```python
from build123d import *

# Parameters (mm, degrees)
BOSS_EXTRUDE1_DEPTH = 40
SKETCH2_R           = 15
BOSS_EXTRUDE2_DEPTH = 12
BOSS_EXTRUDE3_START = 20
SKETCH3_R           = 15
BOSS_EXTRUDE3_DEPTH = 20


with BuildPart() as part:
    # Sketch1 → Boss-Extrude1 (new body)
    with BuildSketch(Plane(origin=(0, 0, 0), x_dir=(1, 0, 0), z_dir=(0, 1, 0))):
        with BuildLine():
            Line((-4, 11), (4, 11))
            Line((4, 11), (4, 14.456832295))
            ThreePointArc((4, 14.456832295), (0, -15), (-4, 14.456832295))
            Line((-4, 14.456832295), (-4, 11))
        make_face()
    extrude(amount=BOSS_EXTRUDE1_DEPTH)

    # Sketch2 → Boss-Extrude2 (add)
    with BuildSketch(Plane(origin=(0, 40, 0), x_dir=(1, 0, 0), z_dir=(0, 1, 0))):
        with Locations(Location((0, 0, 0), (0, 0, 74.533990047))):
            Circle(SKETCH2_R)
    extrude(amount=BOSS_EXTRUDE2_DEPTH)

    # Sketch3 → Boss-Extrude3 (add)
    with BuildSketch(Plane.XZ.offset(BOSS_EXTRUDE3_START)):
        with Locations(Location((0, 0, 0), (0, 0, 270))):
            Circle(SKETCH3_R)
    extrude(amount=-BOSS_EXTRUDE3_DEPTH)


solid = part.part
```
Check sheet for the modelled part. Datum: model origin and axes. Units: mm. Coordinates: 2 decimals unless noted, no trailing zeros. Write each loop counter-clockwise with the first axis right and the second up, starting at its lowest first coordinate (ties: lowest second). Pieces come first, ordered by that corner, then holes. Notation, with made-up numbers: (60.5, 77.25) -> (114.5, 77.25) arc R24 cw to (114.5, 114.25) -> close; hole circle Ø2 at (38, 14). An arc over 180 degrees is marked (long way). Use a Markdown table: item, result.
1. Sectioned sample at B-B (y = 13). Enter the section's corners in (x, z), plus the area to 3 significant figures.
Reported:
| item | result |
|---|---|
| outline | (-4, -14.46) -> (-4, -11) -> (4, -11) -> (4, -14.46) arc R15 ccw (long way) to start |
| area | 676 mm2 |
2. Scan lines: line 1 along Z through (x, y) = (5, 22.5); line 2 along Z through (x, y) = (-7, 44); line 3 along X through (y, z) = (-12.5, 9.75). Record each from-to range of solid material in increasing order.
Reported:
| item | result |
|---|---|
| line 1 | z = -14.14 to 14.14 |
| line 2 | z = -13.27 to 13.27 |
| line 3 | x = -11.4 to 11.4 |
3. Sectioned sample at D-D (y = -6). Enter the section's corners in (x, z), plus the area to 3 significant figures.
Reported:
| item | result |
|---|---|
| outline | circle Ø30 at (0, 0) |
| area | 707 mm2 |
4. Go/stop test with flat-tipped pins: pin 1 Ø1.5 at (x, y) = (-11, 3) entering from -Z; pin 2 Ø4 at (x, y) = (2.5, -12) entering from -Z; pin 3 Ø12 at (x, y) = (11, -13) entering from +Z. Record where each tip stops, or that it passes through.
Reported:
| item | result |
|---|---|
| pin 1 | stops at z = -10.95 |
| pin 2 | stops at z = -14.99 |
| pin 3 | stops at z = 14.14 |
5. Release check for a two-part mould opening along Y. For faces 1 (the flat face through (0, 52, 0)), 2 (the flat face through (0, -20, 0)), 3 (the flat face through (-4, 20, -13)) record: pulls with the +Y half, pulls with the -Y half, needs draft (parallel to the pull), parting line crosses it, or undercut.
Reported:
| item | result |
|---|---|
| face 1 | pulls with the +Y half |
| face 2 | pulls with the -Y half |
| face 3 | undercut |
6. Sectioned sample at A-A (x = 0). Enter the section's corners in (y, z), plus the area to 3 significant figures.
Reported:
| item | result |
|---|---|
| outline | (-20, -15) -> (0, -15) -> (0, -11) -> (40, -11) -> (40, -15) -> (52, -15) -> (52, 15) -> (-20, 15) -> close |
| area | 2,000 mm2 |
7. Sectioned sample at C-C (z = 8.75). Enter the section's corners in (x, y), plus the area to 3 significant figures.
Reported:
| item | result |
|---|---|
| outline | (-12.18, -20) -> (12.18, -20) -> (12.18, 52) -> (-12.18, 52) -> close |
| area | 1,750 mm2 |
